Could you check a few things on this model? Use its own coordinates, in mm. A direction names the side the tool comes from. Round coordinates to 2 decimals unless told otherwise and drop trailing zeros. Loops run counter-clockwise (first coordinate to the right, second up) from the corner with the lowest first, then second, coordinate; pieces in that order, holes last. Notation, with made-up numbers: (-6.5, -2) -> (13.5, -2) arc R25 ccw to (13.5, 18) -> close; hole circle Ø1 at (4.25, 50). An arc over 180 degrees is marked (long way). One line per item, written item: value.
```python
from build123d import *

# Parameters (mm, degrees)
SKETCH2_R         = 0.25
CIRPATTERN1_COUNT = 4


with BuildPart() as part:
    # Sketch1 → Revolve1 (revolve)
    with BuildSketch(Plane(origin=(0, 0, 0), x_dir=(0, 0, -1), z_dir=(1, 0, 0)), mode=Mode.PRIVATE) as revolve1_sk:
        Polygon((-9.925, 0), (-9.7, 16.67), (-8.47, 16.67), (-8.425, 27.08), (-7.39, 27.08), (-7.485, 14.68), (-8.611859628, 14.68), (-8.81, 0), align=None)
    revolve(revolve1_sk.sketch.rotate(Axis((0, 0, 0), (0, 1, 0)), 180), axis=Axis((0, 0, 0), (0, 1, 0)))

    # Sweep1: sweep along a path in Sketch3
    with BuildLine(Plane(origin=(0, 0, 0), x_dir=(0, 0, -1), z_dir=(1, 0, 0))) as sweep1_path:
        Line((8.81, 0), (8.611859628, 14.68))
    # Sketch2 → Sweep1 (sweep)
    with BuildSketch(Plane.XZ):
        with Locations((0, -8.81)):
            Circle(SKETCH2_R)
    sweep1 = sweep(path=sweep1_path.line)

    # CirPattern1: Sweep1 ×4 about axis
    cirpattern1_axis = Axis((0, 0, 0), (0, -1, 0))
    for i in range(1, CIRPATTERN1_COUNT):
        add(sweep1.rotate(cirpattern1_axis, i * 360 / CIRPATTERN1_COUNT))


solid = part.part
```
Item 1: I need wall thicknesses on line 1 (Y direction, x = 7, z = -6.5); line 2 (Z direction, x = 1.75, y = 22.5); line 3 (Z direction, x = 4.25, y = 19.5). Which ranges of each line are inside material? Lowest first, please. Write a range as from..to.
Output:
line 1: y = 0..16.67
line 2: z = -8.26..-7.22, 7.22..8.26
line 3: z = -7.31..-6.12, 6.12..7.31
Item 2: If we section it at A-A on y = 17.5: List the corners of the cut face in (x, z) for me, plus the area to 3 significant figures.
Output:
outline: circle Ø16.93 at (0, 0); hole circle Ø14.93 at (0, 0)
area: 50.2 mm²
Item 3: If we mould it in two halves opening along Z, with no side actions, what happens to faces 1 (the face through (6.23, 7.24, -6.09)), 2 (the face through (-8, 14.68, 0)), 3 (the face through (9, 16.67, 0)), 4 (the face through (9.578, 8.452, 2.127))? For each: released by +Z, released by -Z, zero draft, split by the parting line, or undercut.
Output:
face 1: undercut
face 2: undercut
face 3: zero draft
face 4: split by the parting line
Item 4: For faces 5 (the face through (-6.23, 7.24, 6.09)), 6 (the face through (-9, 0, 0)), 7 (the face through (-2.537, 21.948, -8.057)), which set-ups out of +Z, -Z, +X, -X, +Y, -Y let a thin tool reach every point of the face, with its end or its side?
Output:
face 5: -Y
face 6: +Z, -Z, +X, -X, -Y
face 7: +Y
Item 5: Will these pins go through, and if not, where does the flat tip stop? pin 1 Ø5 at (y, z) = (19.5, -2.5) entering from -X; pin 2 Ø8 at (x, y) = (-3, 18.5) entering from -Z; pin 3 Ø10 at (x, y) = (0.5, 12.5) entering from -Z.
Output:
pin 1: stops at x = -8.46
pin 2: stops at z = -9.71
pin 3: stops at z = -9.82
